Check sheet for the modelled part. Datum: model origin and axes. Units: mm. Face numbers are marked on the shaded views. A direction names the side the tool comes from. Coordinates: 2 decimals unless noted, no trailing zeros. Loops run counter-clockwise (first coordinate to the right, second up) from the corner with the lowest first, then second, coordinate; pieces in that order, holes last. Notation, with made-up numbers: M 56,28.25 L 101,28.25 A15 cw 101,50.25 Z; hole C 79,42.25 d4. An arc over 180 degrees is marked long. Use CSV: the item, a comma, the result in double quotes. Start each with the question number.
(1) Section check B-B on y = -3.75. Record the cut outline in (x, z).
(2) Scan lines: line 1 (Z direction, x = -1.2, y = 2.75); line 2 (X direction, y = 0.25, z = -2.95); line 3 (Y direction, x = -1.45, z = 0.9). Record each from-to range of solid material in increasing order.
(3) Set-up check for the marked faces 1, 2 and 3: record each of +Z, -Z, +X, -X, +Y, -Y from which the full face is reachable in a straight line by a thin tool's end or side.
(4) Section check A-A on x = -0.05. Record the cut outline in (y, z).
(5) Go/stop test with flat-tipped pins: pin 1 Ø0.5 at (y, z) = (0, 0.5) entering from +X; pin 2 Ø1.5 at (x, z) = (-1, -1.5) entering from -Y; pin 3 Ø1 at (x, y) = (-1, -3.5) entering from +Z. Record where each tip stops, or that it passes through.
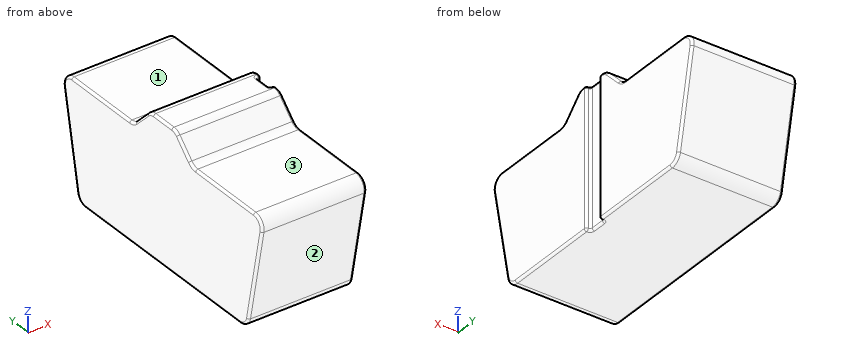
from build123d import *

# Parameters (mm, degrees)
BOSS_EXTRUDE2_START      = -3
BOSS_EXTRUDE2_DEPTH      = 4.5
BOSS_EXTRUDE3_DEPTH      = 1.3
BOSS_EXTRUDE3_DEPTH_BACK = 3
SKETCH2_3_W              = 0.8
SKETCH2_3_H              = 5.98
FILLET1_R                = 0.1


with BuildPart() as part:
    # Sketch2 → Boss-Extrude2 (new body)
    with BuildSketch(Plane.YZ.offset(BOSS_EXTRUDE2_START)):
        with BuildLine():
            Line((-0.4, -3.49), (-0.4, 2.49))
            Line((-0.4, 2.49), (-0.542893219, 2.49))
            ThreePointArc((-0.542893219, 2.49), (-0.730408101, 2.452700971), (-0.889375542, 2.346482323))
            Line((-0.889375542, 2.346482323), (-1.596482323, 1.639375542))
            ThreePointArc((-1.596482323, 1.639375542), (-1.761938231, 1.528821438), (-1.957106781, 1.49))
            Line((-1.957106781, 1.49), (-5.390098049, 1.49))
            ThreePointArc((-5.390098049, 1.49), (-5.769035698, 1.310654564), (-5.87058258, 0.903903094))
            Line((-5.87058258, 0.903903094), (-5.07058258, -3.096096906))
            ThreePointArc((-5.07058258, -3.096096906), (-4.900752612, -3.378937649), (-4.590098049, -3.49))
            Line((-4.590098049, -3.49), (-0.4, -3.49))
        make_face()
    boss_extrude2 = extrude(amount=BOSS_EXTRUDE2_DEPTH)

    # Sketch2<3> → Boss-Extrude3 (add, two sides: drawn at the far end of the back side and taken through both)
    with BuildSketch(Plane.YZ.offset(-BOSS_EXTRUDE3_DEPTH_BACK)):
        with Locations((0, -0.5)):
            Rectangle(SKETCH2_3_W, SKETCH2_3_H)
    extrude(amount=BOSS_EXTRUDE3_DEPTH + BOSS_EXTRUDE3_DEPTH_BACK)

    # Mirror1: Boss-Extrude2 across plane
    add(boss_extrude2.mirror(Plane.ZX))

    # Fillet1
    fillet1_edges = [part.edges().sort_by_distance(p)[0] for p in [
        (1.3, -0.4, -0.5),
        (1.3, 0.4, -0.5),
    ]]
    fillet(fillet1_edges, radius=FILLET1_R)
    fillet1_2_edges = [part.edges().sort_by_distance(p)[0] for p in [
        (1.3, 0, -3.49),
        (1.3, 0, 2.49),
        (1.5, 5.769035698, 1.310654564),
        (1.5, 5.47058258, -1.096096906),
        (1.5, 4.900752612, -3.378937649),
        (1.5, 2.495049024, -3.49),
        (1.5, 0.4, -0.5),
        (1.5, 0.471446609, 2.49),
        (1.5, 0.730408101, 2.452700971),
        (1.5, 1.242928932, 1.992928932),
        (1.5, 1.761938231, 1.528821438),
        (1.5, 3.673602415, 1.49),
        (1.5, -1.761938231, 1.528821438),
        (1.5, -1.242928932, 1.992928932),
        (1.5, -0.730408101, 2.452700971),
        (1.5, -0.471446609, 2.49),
        (1.5, -0.4, -0.5),
        (1.5, -2.495049024, -3.49),
        (1.5, -4.900752612, -3.378937649),
        (1.5, -5.47058258, -1.096096906),
        (1.5, -5.769035698, 1.310654564),
        (1.5, -3.673602415, 1.49),
        (-3, -5.769035698, 1.310654564),
        (-3, -5.47058258, -1.096096906),
        (-3, -4.900752612, -3.378937649),
        (-3, 0, -3.49),
        (-3, 4.900752612, -3.378937649),
        (-3, 5.47058258, -1.096096906),
        (-3, 5.769035698, 1.310654564),
        (-3, 3.673602415, 1.49),
        (-3, 1.761938231, 1.528821438),
        (-3, 1.242928932, 1.992928932),
        (-3, 0.730408101, 2.452700971),
        (-3, 0, 2.49),
        (-3, -0.730408101, 2.452700971),
        (-3, -1.242928932, 1.992928932),
        (-3, -1.761938231, 1.528821438),
        (-3, -3.673602415, 1.49),
        (1.329289322, 0.370710678, 2.49),
        (1.329289322, -0.370710678, 2.49),
        (1.329289322, -0.370710678, -3.49),
        (1.329289322, 0.370710678, -3.49),
    ]]
    fillet(fillet1_2_edges, radius=FILLET1_R - 0.0001)  # a hair under: the kernel refuses the full size


solid = part.part
Outcome:
1,outline,"M -3,-3.39 A0.1 ccw -2.9,-3.49 L 1.4,-3.49 A0.1 ccw 1.5,-3.39 L 1.5,1.39 A0.1 ccw 1.4,1.49 L -2.9,1.49 A0.1 ccw -3,1.39 Z"
2,line 1,"z = -3.49 to 1.49"
2,line 2,"x = -3 to 1.3"
2,line 3,"y = -5.87 to 5.87"
3,face 1,"+Z, +X, -X, +Y"
3,face 2,"-Z, +X, -X, -Y"
3,face 3,"+Z, +X, -X, -Y"
4,outline,"M -5.87,0.9 L -5.07,-3.1 A0.49 ccw -4.59,-3.49 L 4.59,-3.49 A0.49 ccw 5.07,-3.1 L 5.87,0.9 A0.49 ccw 5.39,1.49 L 1.96,1.49 A0.51 cw 1.6,1.64 L 0.89,2.35 A0.49 ccw 0.54,2.49 L -0.54,2.49 A0.49 ccw -0.89,2.35 L -1.6,1.64 A0.51 cw -1.96,1.49 L -5.39,1.49 A0.49 ccw Z"
5,pin 1,"stops at x = 1.3"
5,pin 2,"stops at y = -5.54"
5,pin 3,"stops at z = 1.49"
